from build123d import *

# Parameters (mm, degrees)
SKETCH1_W           = 203.029806175
SKETCH1_H           = 31.75
BOSS_EXTRUDE1_DEPTH = 6.35
CUT_EXTRUDE1_REACH  = 241.441
SKETCH2_W           = 19.829806175
SKETCH2_H           = 6.35
SKETCH2_W_2         = 50.8
SKETCH2_W_3         = 30.8


with BuildPart() as part:
    # Sketch1 → Boss-Extrude1 (new body)
    with BuildSketch(Plane.XY):
        with Locations((132.485096913, 34.478439237)):
            Rectangle(SKETCH1_W, SKETCH1_H)
    extrude(amount=BOSS_EXTRUDE1_DEPTH)

    # Sketch2 → Cut-Extrude1 (cut, up to next)
    with BuildSketch(Plane.XY.offset(6.35), mode=Mode.PRIVATE) as cut_extrude1_sk1:
        with Locations((40.885096913, 21.778439237)):
            Rectangle(SKETCH2_W, SKETCH2_H)
    cut_extrude1_tool1 = extrude(cut_extrude1_sk1.sketch, amount=-CUT_EXTRUDE1_REACH, mode=Mode.PRIVATE) & part.part
    # Sketch2 → Cut-Extrude1 (cut, up to next)
    with BuildSketch(Plane.XY.offset(6.35), mode=Mode.PRIVATE) as cut_extrude1_sk2:
        with Locations((127, 21.778439237)):
            Rectangle(SKETCH2_W_2, SKETCH2_H)
    cut_extrude1_tool2 = extrude(cut_extrude1_sk2.sketch, amount=-CUT_EXTRUDE1_REACH, mode=Mode.PRIVATE) & part.part
    # Sketch2 → Cut-Extrude1 (cut, up to next)
    with BuildSketch(Plane.XY.offset(6.35), mode=Mode.PRIVATE) as cut_extrude1_sk3:
        with Locations((218.6, 21.778439237)):
            Rectangle(SKETCH2_W_3, SKETCH2_H)
    cut_extrude1_tool3 = extrude(cut_extrude1_sk3.sketch, amount=-CUT_EXTRUDE1_REACH, mode=Mode.PRIVATE) & part.part
    add(cut_extrude1_tool1.solids().sort_by_distance((40.885097, 21.778439, 6.35))[0], mode=Mode.SUBTRACT)
    add(cut_extrude1_tool2.solids().sort_by_distance((127, 21.778439, 6.35))[0], mode=Mode.SUBTRACT)
    add(cut_extrude1_tool3.solids().sort_by_distance((218.6, 21.778439, 6.35))[0], mode=Mode.SUBTRACT)


solid = part.part
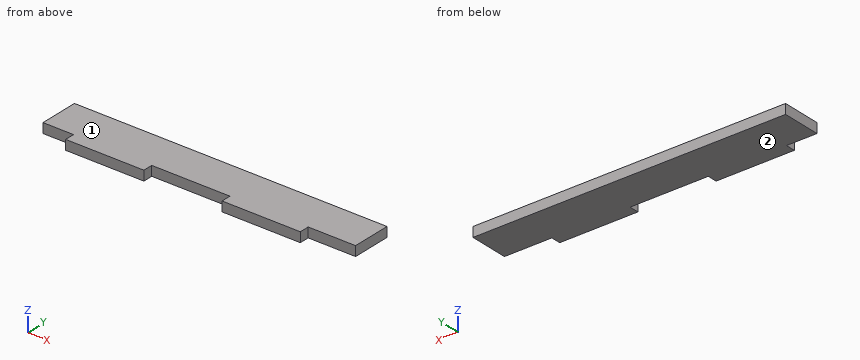
Could you check a few things on this model? Use its own coordinates, in mm. Face numbers are marked on the shaded views. Coordinates: 2 decimals unless noted, no trailing zeros. Order: outer loops, then holes, each group sorted by start corner. A loop starts at its lowest first (then second) coordinate and runs counter-clockwise, first axis right, second up. Notation, with made-up numbers: (51, 80) - (69, 80) arc R12 cw to (69, 88) - close; hole circle Ø7 at (-13, 63). An arc over 180 degrees is marked (long way). Answer in a Markdown table with one row per item. Add a question column.
(1) If we section it at B-B, the plane z = 1: Please give me the cut outline in (x, y), then the cut area to 3 significant figures.
(2) Will this pin go through, and if not, where does the flat tip stop? pin 1 (1.9 mm diameter, centred on x = 45, z = 4.5, fed in from -Y).
(3) I need wall thicknesses on L1, parallel to X at y = 22, z = 2.75; L2, parallel to Y at x = 104.5, z = 6. Which ranges of each line are inside material? Lowest first, please.
(4) If we section it at A-A, the plane y = 22.5: Please give me the cut outline in (x, z).
(5) If we section it at C-C, the plane x = 123: Please give me the cut outline in (y, z), then the cut area to 3 significant figures.
(6) If we mould it in two halves opening along Z, with no side actions, what happens to the marked faces 1 and 2? For each: released by +Z, released by -Z, zero draft, split by the parting line, or undercut.
Results are:
| question | item | result |
|---|---|---|
| 1 | outline | (30.97, 24.95) - (50.8, 24.95) - (50.8, 18.6) - (101.6, 18.6) - (101.6, 24.95) - (152.4, 24.95) - (152.4, 18.6) - (203.2, 18.6) - (203.2, 24.95) - (234, 24.95) - (234, 50.35) - (30.97, 50.35) - close |
| 1 | area | 5,800 mm2 |
| 2 | pin 1 | stops at y = 24.95 |
| 3 | L1 | x = 50.8 to 101.6, 152.4 to 203.2 |
| 3 | L2 | y = 24.95 to 50.35 |
| 4 | outline | (50.8, 0) - (101.6, 0) - (101.6, 6.35) - (50.8, 6.35) - close; (152.4, 0) - (203.2, 0) - (203.2, 6.35) - (152.4, 6.35) - close |
| 5 | outline | (24.95, 0) - (50.35, 0) - (50.35, 6.35) - (24.95, 6.35) - close |
| 5 | area | 161 mm2 |
| 6 | face 1 | released by +Z |
| 6 | face 2 | released by -Z |
